Source: three-view drawing plus pictorial views. Frame: mm from the lowest corner of the part. A direction names the side the tool comes from. Give positions to 0.01 mm unless a question says otherwise; leave off trailing zeros. Order: outer loops, then holes, each group sorted by start corner. A loop starts at its lowest first (then second) coordinate and runs counter-clockwise, first axis right, second up. Notation, with made-up numbers: (49, -35.5) - (100, -35.5) arc R19 cw to (100, -21.5) - close; hole circle Ø11 at (11, -30). An arc over 180 degrees is marked (long way). Answer in a Markdown table with one row per item. Add a question column.
1. Section query B-B on z = 18. Return loops of the section in (x, y).
2. Contact query for flat-ended pins moving along their axis: pin 1 (4 mm diameter, centred on x = 59.5, y = 71, fed in from -Z); pin 2 (2.5 mm diameter, centred on x = 20, z = 18, fed in from +Y); pin 3 (5.5 mm diameter, centred on y = 3.5, z = 18.5, fed in from +X); pin 4 (2.5 mm diameter, centred on y = 114, z = 13, fed in from -X). Output: stop coordinate, or through.
3. Section query C-C on x = 20. Return loops of the section in (y, z).
4. Section query A-A on x = 72. Return loops of the section in (y, z), and give its area (4 significant figures).
5. Access query for the marked faces 4 and 5. Directions: +Z, -Z, +X, -X, +Y, -Y. A direction counts if a zero-diameter tool reaches every point of the face in a straight line with its end or side. Return the directions, or none.
6. Section query D-D on z = 6.25. Return loops of the section in (x, y).
7. Mould query, pull axis Y, two halves, no side actions, for the marked faces 1, 2 and 3. Classes: released by +Y, released by -Y, zero draft, split by the parting line, or undercut.
8. Ray query, line 1 (X direction, y = 3.55, z = 18); line 2 (X direction, y = 113, z = 18); line 3 (Z direction, x = 72, y = 114). Return the intervals inside material, ascending. Write a range as [from, to].
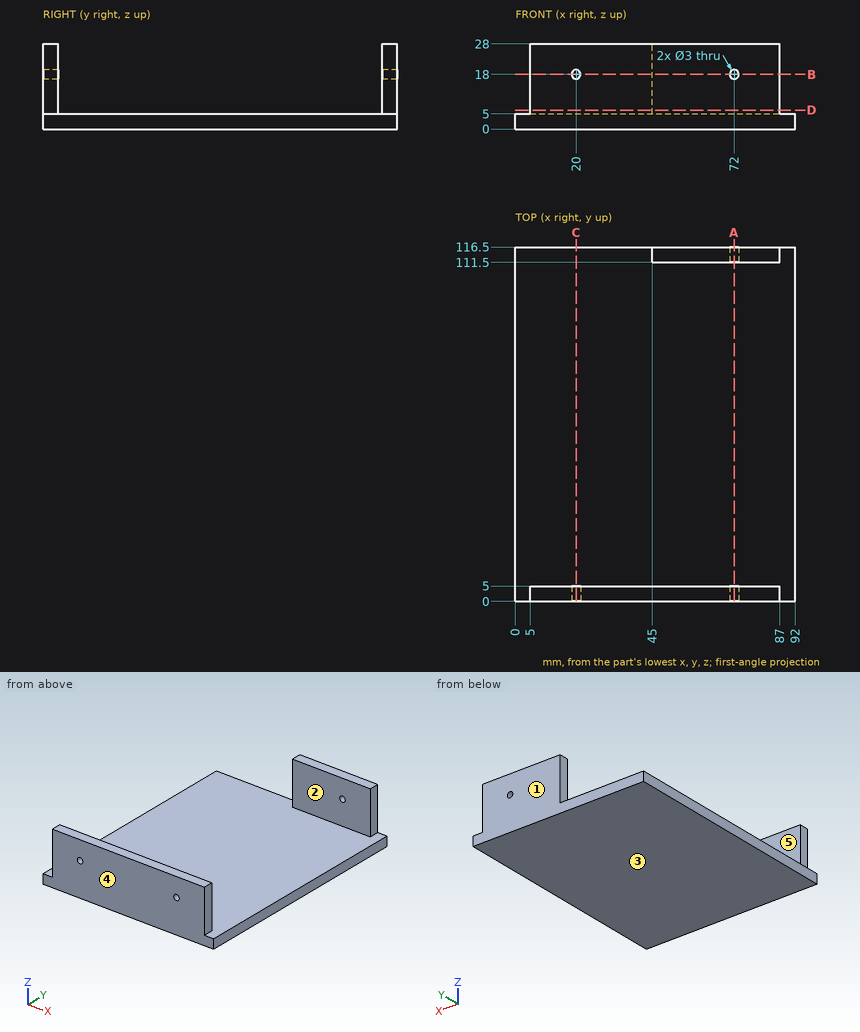
Answer:
| question | item | result |
|---|---|---|
| 1 | outline | (5, 0) - (18.5, 0) - (18.5, 5) - (5, 5) - close; (21.5, 0) - (70.5, 0) - (70.5, 5) - (21.5, 5) - close; (45, 111.5) - (70.5, 111.5) - (70.5, 116.5) - (45, 116.5) - close; (73.5, 0) - (87, 0) - (87, 5) - (73.5, 5) - close; (73.5, 111.5) - (87, 111.5) - (87, 116.5) - (73.5, 116.5) - close |
| 2 | pin 1 | stops at z = 0 |
| 2 | pin 2 | passes through |
| 2 | pin 3 | stops at x = 87 |
| 2 | pin 4 | stops at x = 45 |
| 3 | outline | (0, 0) - (116.5, 0) - (116.5, 5) - (5, 5) - (5, 16.5) - (0, 16.5) - close; (0, 19.5) - (5, 19.5) - (5, 28) - (0, 28) - close |
| 4 | outline | (0, 0) - (116.5, 0) - (116.5, 16.5) - (111.5, 16.5) - (111.5, 5) - (5, 5) - (5, 16.5) - (0, 16.5) - close; (0, 19.5) - (5, 19.5) - (5, 28) - (0, 28) - close; (111.5, 19.5) - (116.5, 19.5) - (116.5, 28) - (111.5, 28) - close |
| 4 | area | 782.5 mm² |
| 5 | face 4 | +Z, -Z, +X, -X, -Y |
| 5 | face 5 | +Z, +X, -X |
| 6 | outline | (5, 0) - (87, 0) - (87, 5) - (5, 5) - close; (45, 111.5) - (87, 111.5) - (87, 116.5) - (45, 116.5) - close |
| 7 | face 1 | released by +Y |
| 7 | face 2 | undercut |
| 7 | face 3 | zero draft |
| 8 | line 1 | x = [5, 18.5], [21.5, 70.5], [73.5, 87] |
| 8 | line 2 | x = [45, 70.5], [73.5, 87] |
| 8 | line 3 | z = [0, 16.5], [19.5, 28] |
